```python
from build123d import *

# Parameters (mm, degrees)
SKETCH011_W     = 81
SKETCH011_H     = 41
PAD002_DEPTH    = 2
SKETCH012_W     = 79
SKETCH012_H     = 39
PAD003_DEPTH    = 12
SKETCH059_W     = 77
SKETCH059_H     = 37
POCKET022_DEPTH = 12
SKETCH060_W     = 30
SKETCH060_H     = 2
POCKET023_DEPTH = 2
SKETCH061_W     = 24
SKETCH061_H     = 11.75
POCKET024_DEPTH = 2
SKETCH103_W     = 10
SKETCH103_H     = 11.75
POCKET038_DEPTH = 2
SKETCH104_W     = 10
SKETCH104_H     = 11.75
POCKET039_DEPTH = 2


with BuildPart() as part:
    # Sketch011 (on DatumPlane) → Pad002 (new body)
    with BuildSketch(Plane(origin=(0, 0, 0), x_dir=(1, 0, 0), z_dir=(0, 1, 0))):
        Rectangle(SKETCH011_W, SKETCH011_H)
    extrude(amount=-PAD002_DEPTH)

    # Sketch012 → Pad003 (join)
    with BuildSketch(Plane.XZ.offset(1.75)):
        Rectangle(SKETCH012_W, SKETCH012_H)
    extrude(amount=PAD003_DEPTH)

    # Sketch059 (on Face11 of Pad003) → Pocket022 (cut)
    with BuildSketch(Plane.XZ.offset(13.75)):
        Rectangle(SKETCH059_W, SKETCH059_H)
    extrude(amount=-POCKET022_DEPTH, mode=Mode.SUBTRACT)

    # Sketch060 (on Face4 of Pocket022) → Pocket023 (cut)
    with BuildSketch(Plane(origin=(0, 0, 0), x_dir=(1, 0, 0), z_dir=(0, 1, 0))):
        with Locations((18.5, -10)):
            Rectangle(SKETCH060_W, SKETCH060_H)
        with Locations((18.5, -5)):
            Rectangle(SKETCH060_W, SKETCH060_H)
        with Locations((18.5, 0)):
            Rectangle(SKETCH060_W, SKETCH060_H)
        with Locations((18.5, 5)):
            Rectangle(SKETCH060_W, SKETCH060_H)
        with Locations((18.5, 10)):
            Rectangle(SKETCH060_W, SKETCH060_H)
        with Locations((-18.5, -10)):
            Rectangle(SKETCH060_W, SKETCH060_H)
        with Locations((-18.5, -5)):
            Rectangle(SKETCH060_W, SKETCH060_H)
        with Locations((-18.5, 0)):
            Rectangle(SKETCH060_W, SKETCH060_H)
        with Locations((-18.5, 5)):
            Rectangle(SKETCH060_W, SKETCH060_H)
        with Locations((-18.5, 10)):
            Rectangle(SKETCH060_W, SKETCH060_H)
    extrude(amount=-POCKET023_DEPTH, mode=Mode.SUBTRACT)

    # Sketch061 (on Face50 of Pocket023) → Pocket024 (cut)
    with BuildSketch(Plane(origin=(0, 0, -19.5), x_dir=(-1, 0, 0), z_dir=(0, 0, -1))):
        with Locations((-3, -7.875)):
            Rectangle(SKETCH061_W, SKETCH061_H)
    extrude(amount=-POCKET024_DEPTH, mode=Mode.SUBTRACT)

    # Sketch103 (on Face1 of Pocket024) → Pocket038 (cut)
    with BuildSketch(Plane.ZY.offset(39.5)):
        with Locations((4, -7.875)):
            Rectangle(SKETCH103_W, SKETCH103_H)
    extrude(amount=-POCKET038_DEPTH, mode=Mode.SUBTRACT)

    # Sketch104 (on Face15 of Pocket038) → Pocket039 (cut)
    with BuildSketch(Plane(origin=(39.5, 0, 0), x_dir=(0, 0, -1), z_dir=(1, 0, 0))):
        with Locations((-4, -7.875)):
            Rectangle(SKETCH104_W, SKETCH104_H)
    extrude(amount=-POCKET039_DEPTH, mode=Mode.SUBTRACT)


solid = part.part
```
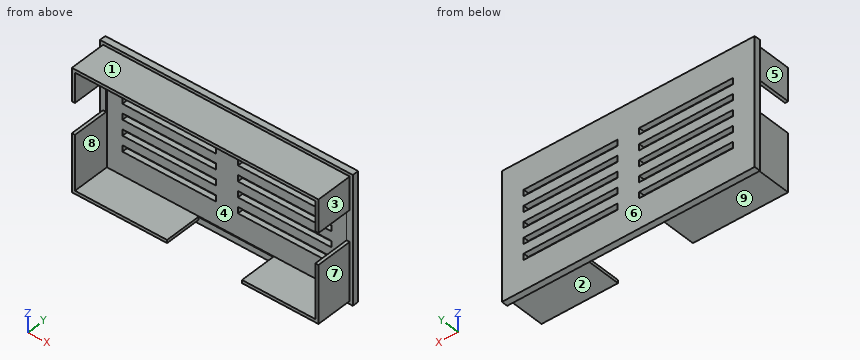
Could you check a few things on this model? Use its own coordinates, in mm. Face numbers are marked on the shaded views. A direction names the side the tool comes from. Coordinates: 2 decimals unless noted, no trailing zeros. Loops run counter-clockwise (first coordinate to the right, second up) from the corner with the lowest first, then second, coordinate; pieces in that order, holes last.
1) Which directions (+Z, -Z, +X, -X, +Y, -Y) give clear straight access to the entire face, cutting with the end or side of a thin tool? Please do the marked faces 5, 6, 7, 8 and 9.
Reported:
face 5: +Z, -Z, -X, -Y
face 6: +Z, -Z, +X, -X, +Y
face 7: +Z, -Z, +X, -Y
face 8: -Y
face 9: -Z, +X, -X, -Y
2) Please list where these lines run through material, in increasing order: line 1 along Z through (x, y) = (-12, -0.5); line 2 along X through (y, z) = (-1.5, -10.5); line 3 along Z through (x, y) = (-20, -7).
Reported:
line 1: z = -20.5 to -11, -9 to -6, -4 to -1, 1 to 4, 6 to 9, 11 to 20.5
line 2: x = -40.5 to -33.5, -3.5 to 3.5, 33.5 to 40.5
line 3: z = -19.5 to -18.5, 18.5 to 19.5
3) Will these pins go through, and if not, where does the flat tip stop? pin 1 Ø20.5 at (x, z) = (0, -6.5) entering from -Y; pin 2 Ø2 at (x, y) = (17.5, -4.5) entering from -Z; pin 3 Ø6 at (x, y) = (-16.5, -10) entering from +Z; pin 4 Ø1 at (x, z) = (-9.5, 0) entering from +Y.
Reported:
pin 1: stops at y = -1.75
pin 2: stops at z = -19.5
pin 3: stops at z = 19.5
pin 4: passes through
4) Thinking about a two-plate mould opening in Z: for the marked faces 1, 2, 3 and 4, which applies, released by +Z, released by -Z, zero draft, split by the parting line, or undercut?
Reported:
face 1: released by +Z
face 2: released by -Z
face 3: zero draft
face 4: undercut
5) Imagine slicing it at A-A (x = -32). State how many separate pieces and enclosed holes the cut face has, and give its area (4 significant figures).
Reported:
separate pieces: 6
enclosed holes: 0
area: 78.75 mm2
6) Imagine slicing it at C-C (z = -13). List the corners of the cut face in (x, y) for me.
Reported:
outline: (-40.5, -2) - (-39.5, -2) - (-39.5, -13.75) - (-38.5, -13.75) - (-38.5, -1.75) - (38.5, -1.75) - (38.5, -13.75) - (39.5, -13.75) - (39.5, -2) - (40.5, -2) - (40.5, 0) - (-40.5, 0) - close
7) Imagine slicing it at B-B (y = -6). List the corners of the cut face in (x, z) for me, and give its area (3 significant figures).
Reported:
outline: (-39.5, -19.5) - (-9, -19.5) - (-9, -18.5) - (-38.5, -18.5) - (-38.5, -1) - (-39.5, -1) - close; (-39.5, 9) - (-38.5, 9) - (-38.5, 18.5) - (38.5, 18.5) - (38.5, 9) - (39.5, 9) - (39.5, 19.5) - (-39.5, 19.5) - close; (15, -19.5) - (39.5, -19.5) - (39.5, -1) - (38.5, -1) - (38.5, -18.5) - (15, -18.5) - close
area: 188 mm2
